Design review of the part built by this model. Coordinates are the model's own, in mm. A direction names the side the tool comes from. Give positions to 0.01 mm unless a question says otherwise; leave off trailing zeros. Order: outer loops, then holes, each group sorted by start corner. A loop starts at its lowest first (then second) coordinate and runs counter-clockwise, first axis right, second up. Notation, with made-up numbers: (58.25, 5.25) -> (110.25, 5.25) arc R20 ccw to (110.25, 14.25) -> close; hole circle Ø4 at (68, 70). An arc over 180 degrees is marked (long way). Return JSON: item names as keys, results as strings.
```python
from build123d import *

# Parameters (mm, degrees)
SKETCH1_R           = 1.65
BOSS_EXTRUDE1_DEPTH = 3.175


with BuildPart() as part:
    # Sketch1 → Boss-Extrude1 (new body)
    with BuildSketch(Plane.XY):
        Polygon((-14, 13.175), (-14, 10), (-14, -10), (-14, -13.175), (-6, -13.175), (-6, -10), (-10, -10), (-10, -6), (10, -6), (10, -10), (6, -10), (6, -13.175), (14, -13.175), (14, -10), (14, 10), (14, 13.175), (6, 13.175), (6, 10), (-6, 10), (-6, 13.175), align=None)
        with Locations((-7.5, 6.7)):
            Circle(SKETCH1_R, mode=Mode.SUBTRACT)
        with Locations((7.5, 6.7)):
            Circle(SKETCH1_R, mode=Mode.SUBTRACT)
    extrude(amount=BOSS_EXTRUDE1_DEPTH)


solid = part.part
```
Item 1: Wall thickness on L1, parallel to Y at x = -7.5, z = 2.4 (3 decimals); L2, parallel to X at y = -12, z = 1.45; L3, parallel to X at y = -9.25, z = 2.75: over which ranges is each line inside the solid? List them lowest first. Write a range as [from, to].
Result set:
{"L1": "y = [-13.175, -10], [-6, 5.05], [8.35, 13.175]", "L2": "x = [-14, -6], [6, 14]", "L3": "x = [-14, -10], [10, 14]"}
Item 2: Add section A-A (y = 6.7). Give the boundary of the cut face in (x, z) (3 decimals), plus the area to 3 significant figures.
Result set:
{"outline": "(-14, 0) -> (-9.15, 0) -> (-9.15, 3.175) -> (-14, 3.175) -> close; (-5.85, 0) -> (5.85, 0) -> (5.85, 3.175) -> (-5.85, 3.175) -> close; (9.15, 0) -> (14, 0) -> (14, 3.175) -> (9.15, 3.175) -> close", "area": "67.9 mm^2"}
Item 3: Add section B-B (z = 0.9). Give the boundary of the cut face in (x, y) (3 decimals), plus the area to 3 significant figures.
Result set:
{"outline": "(-14, -13.175) -> (-6, -13.175) -> (-6, -10) -> (-10, -10) -> (-10, -6) -> (10, -6) -> (10, -10) -> (6, -10) -> (6, -13.175) -> (14, -13.175) -> (14, 13.175) -> (6, 13.175) -> (6, 10) -> (-6, 10) -> (-6, 13.175) -> (-14, 13.175) -> close; hole circle Ø3.3 at (-7.5, 6.7); hole circle Ø3.3 at (7.5, 6.7)", "area": "564 mm^2"}
Item 4: Add section D-D (x = -3.75). Give the boundary of the cut face in (y, z) (3 decimals).
Result set:
{"outline": "(-6, 0) -> (10, 0) -> (10, 3.175) -> (-6, 3.175) -> close"}
Item 5: Mouldability with a two-part tool opening along X and no side actions: class faces 1 (the face through (-10, 13.175, 2)), 2 (the face through (6.284, 7.815, 1.565)), 3 (the face through (14, 0, 2)) as released by +X, released by -X, zero draft, split by the parting line, or undercut.
Result set:
{"face 1": "zero draft", "face 2": "undercut", "face 3": "released by +X"}
Item 6: Add section C-C (x = -7.5). Give the boundary of the cut face in (y, z) (3 decimals), plus the area to 3 significant figures.
Result set:
{"outline": "(-13.175, 0) -> (-10, 0) -> (-10, 3.175) -> (-13.175, 3.175) -> close; (-6, 0) -> (5.05, 0) -> (5.05, 3.175) -> (-6, 3.175) -> close; (8.35, 0) -> (13.175, 0) -> (13.175, 3.175) -> (8.35, 3.175) -> close", "area": "60.5 mm^2"}
Item 7: Machinability: for faces 4 (the face through (10, 13.175, 2)), 5 (the face through (6, -12, 2)), 6 (the face through (6, 12, 2)), 7 (the face through (10, -8, 2)), 8 (the face through (10, -13.175, 2)), which of the approach directions +Z, -Z, +X, -X, +Y, -Y give a long, thin tool a straight path to every point of the face, cutting with its end or side? Answer none if there is none.
Result set:
{"face 4": "+Z, -Z, +X, -X, +Y", "face 5": "+Z, -Z, -Y", "face 6": "+Z, -Z, +Y", "face 7": "+Z, -Z", "face 8": "+Z, -Z, +X, -X, -Y"}
